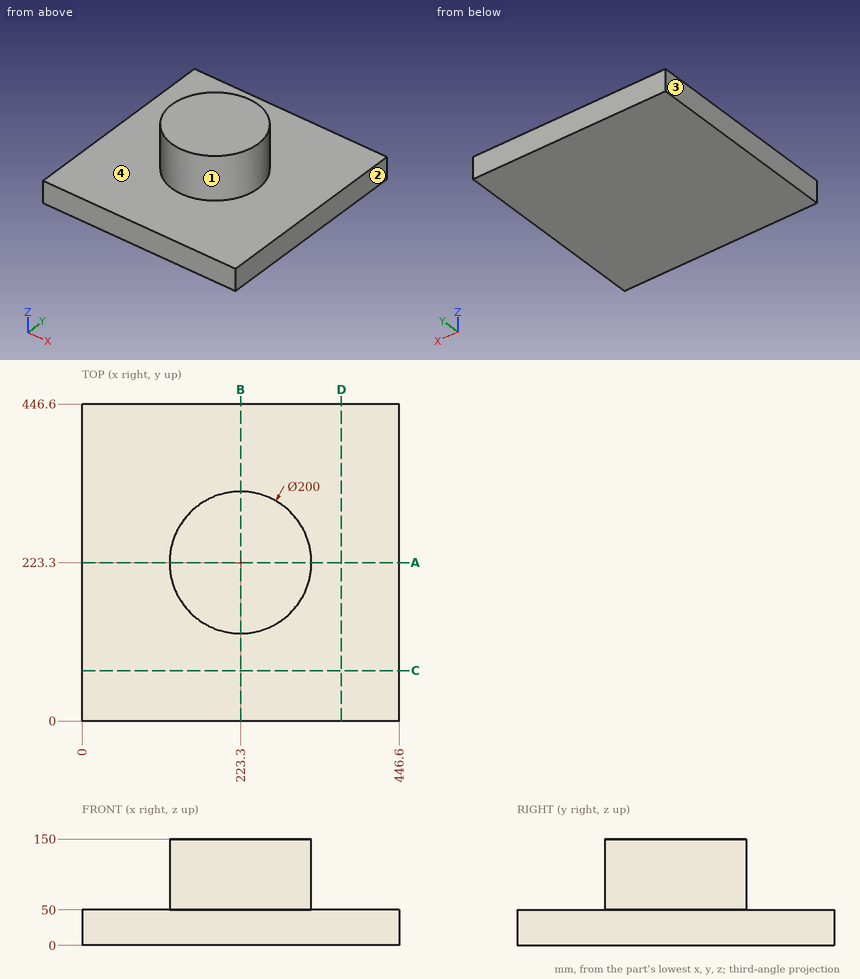
Study the drawing (mm; zero at the part's minimum x, y, z) and answer. Round coordinates to 2 decimals unless told otherwise and drop trailing zeros. Write each loop counter-clockwise with the first axis right and the second up, starting at its lowest first coordinate (ties: lowest second). Pieces come first, ordered by that corner, then holes. Notation, with made-up numbers: (-35, 34) - (2, 34) arc R23 cw to (2, 66) - close; hole circle Ø4 at (10.25, 89.25). An arc over 180 degrees is marked (long way). Use CSV: the item, a comma, the result in double quotes.
Q1. Find section C-C, the plane y = 71. Write down the section's boundary in (x, z).
Values:
outline,"(0, 0) - (446.6, 0) - (446.6, 50) - (0, 50) - close"
Q2. Find section A-A, the plane y = 223.3. Write down the section's boundary in (x, z).
Values:
outline,"(0, 0) - (446.6, 0) - (446.6, 50) - (323.3, 50) - (323.3, 150) - (123.3, 150) - (123.3, 50) - (0, 50) - close"
Q3. Determine the mould class of the marked faces 1, 2, 3 and 4 for opening direction X: +X half, -X half, draft (parallel to the pull), parting line (faces both ways), or undercut.
Values:
face 1,"parting line"
face 2,"+X half"
face 3,"-X half"
face 4,"draft"
Q4. Straight lines are drawn through the part: line 1 along Z through (x, y) = (194, 106.5); line 2 along Y through (x, z) = (245.5, 63); line 3 along Y through (x, z) = (265, 110). For each, find the intervals that lie inside material, in ascending order.
Values:
line 1,"z = 0 to 50"
line 2,"y = 125.8 to 320.8"
line 3,"y = 132.41 to 314.19"
Q5. This flat-tipped pin is pushed along its axis until it touches: pin 1 Ø2 at (y, z) = (142, 76.5) entering from +X. Where does it stop, or does it pass through?
Values:
pin 1,"stops at x = 282.9"
